from build123d import *

# Parameters (mm, degrees)
SKETCH2_R           = 1.5
SKETCH2_R_2         = 1.6
BOSS_EXTRUDE2_DEPTH = 4.25


with BuildPart() as part:
    # Sketch2 → Boss-Extrude2 (new body)
    with BuildSketch(Plane(origin=(0, 0, 0), x_dir=(1, 0, 0), z_dir=(0, 1, 0))):
        Polygon((184.400116, 296), (225.400116, 255), (241.514718626, 255), (282.514718626, 296), (287.485169777, 296), (291, 292.485169777), (291, 287.514718626), (253, 249.514718626), (253, 226.666961), (291, 188.666961), (291, 181.333039), (253, 143.333039), (253, 120.485281374), (291, 82.485281374), (291, 77.514830223), (287.485169777, 74), (282.514718626, 74), (241.514718626, 115), (225.400116, 115), (184.400116, 74), (175.599884, 74), (134.599884, 115), (113.485281374, 115), (72.485281374, 74), (67.514830223, 74), (64, 77.514830223), (64, 82.485281374), (91, 109.485281374), (91, 123), (81.5, 132.5), (81.5, 163.760895), (64, 181.260895), (64, 188.739105), (81.5, 206.239105), (81.5, 237.5), (91, 247), (91, 260.514718626), (64, 287.514718626), (64, 292.485169777), (67.514830223, 296), (72.485281374, 296), (113.485281374, 255), (134.599884, 255), (175.599884, 296), align=None)
        with Locations(Location((180, 80, 0), (0, 0, 270))):
            Circle(SKETCH2_R, mode=Mode.SUBTRACT)
        with Locations(Location((180, 290, 0), (0, 0, 270))):
            Circle(SKETCH2_R, mode=Mode.SUBTRACT)
        with Locations(Location((285, 80, 0), (0, 0, 270))):
            Circle(SKETCH2_R, mode=Mode.SUBTRACT)
        with Locations(Location((70, 290, 0), (0, 0, 270))):
            Circle(SKETCH2_R, mode=Mode.SUBTRACT)
        with Locations(Location((285, 290, 0), (0, 0, 270))):
            Circle(SKETCH2_R, mode=Mode.SUBTRACT)
        with Locations(Location((70, 185, 0), (0, 0, 270))):
            Circle(SKETCH2_R, mode=Mode.SUBTRACT)
        with Locations(Location((180, 185, 0), (0, 0, 270))):
            Circle(SKETCH2_R, mode=Mode.SUBTRACT)
        with Locations(Location((285, 185, 0), (0, 0, 270))):
            Circle(SKETCH2_R, mode=Mode.SUBTRACT)
        with Locations(Location((256.5, 185, 0), (0, 0, 270))):
            Circle(SKETCH2_R_2, mode=Mode.SUBTRACT)
        with Locations(Location((276.5, 185, 0), (0, 0, 270))):
            Circle(SKETCH2_R_2, mode=Mode.SUBTRACT)
        with Locations(Location((106.5, 220, 0), (0, 0, 270))):
            Circle(SKETCH2_R_2, mode=Mode.SUBTRACT)
        with Locations(Location((106.5, 150, 0), (0, 0, 270))):
            Circle(SKETCH2_R_2, mode=Mode.SUBTRACT)
        with Locations(Location((86.5, 220, 0), (0, 0, 270))):
            Circle(SKETCH2_R_2, mode=Mode.SUBTRACT)
        with Locations(Location((86.5, 150, 0), (0, 0, 270))):
            Circle(SKETCH2_R_2, mode=Mode.SUBTRACT)
        with Locations(Location((70, 80, 0), (0, 0, 270))):
            Circle(SKETCH2_R, mode=Mode.SUBTRACT)
        with Locations(Location((181.5, 165.5, 0), (0, 0, 270))):
            Circle(SKETCH2_R, mode=Mode.SUBTRACT)
        with Locations(Location((181.5, 204.5, 0), (0, 0, 270))):
            Circle(SKETCH2_R, mode=Mode.SUBTRACT)
        Polygon((162, 177.02296782), (141.97703218, 157), (124.999970007, 157), (101.5, 180.5), (101.5, 189.5), (124.999970007, 213), (141.97703218, 213), (162, 192.97703218), align=None, mode=Mode.SUBTRACT)
        Polygon((251.5, 210.014709), (240.98529, 220.529449), (224.014709, 220.529449), (197, 193.51474), (197, 176.48526), (224.014709, 149.470551), (240.98529, 149.470551), (251.5, 159.985291), align=None, mode=Mode.SUBTRACT)
        Polygon((143, 246.415771), (143, 229.566314), (159.566314, 213), (199.51474, 213), (216, 229.48526), (216, 247.429580116), (183.682617, 279.746963116), (176.317383, 279.733154), align=None, mode=Mode.SUBTRACT)
        Polygon((143, 123.584229), (143, 140.433686), (159.566314, 157), (199.51474, 157), (216, 140.51474), (216, 122.570419884), (183.682617, 90.253036884), (176.317383, 90.266846), align=None, mode=Mode.SUBTRACT)
        with BuildLine():
            Line((101.500000013, 226.75), (101.500000013, 213.25))
            Line((101.500000013, 213.25), (102.000000013, 212.75))
            Line((102.000000013, 212.75), (102.100000157, 212.75))
            ThreePointArc((102.100000157, 212.75), (105.1, 209.75), (102.100000157, 206.75))
            Line((102.100000157, 206.75), (90.899999843, 206.75))
            ThreePointArc((90.899999843, 206.75), (87.9, 209.75), (90.899999843, 212.75))
            Line((90.899999843, 212.75), (90.999999987, 212.75))
            Line((90.999999987, 212.75), (91.499999987, 213.25))
            Line((91.499999987, 213.25), (91.499999987, 226.75))
            Line((91.499999987, 226.75), (90.999999987, 227.25))
            Line((90.999999987, 227.25), (90.899999843, 227.25))
            ThreePointArc((90.899999843, 227.25), (87.9, 230.25), (90.899999843, 233.25))
            Line((90.899999843, 233.25), (102.100000157, 233.25))
            ThreePointArc((102.100000157, 233.25), (105.100000157, 230.25), (102.100000157, 227.25))
            Line((102.100000157, 227.25), (102.000000013, 227.25))
            Line((102.000000013, 227.25), (101.500000013, 226.75))
        make_face(mode=Mode.SUBTRACT)
        with BuildLine():
            Line((271.500000013, 191.75), (271.500000013, 178.25))
            Line((271.500000013, 178.25), (272.000000013, 177.75))
            Line((272.000000013, 177.75), (272.100000157, 177.75))
            ThreePointArc((272.100000157, 177.75), (275.100000157, 174.75), (272.100000157, 171.75))
            Line((272.100000157, 171.75), (260.899999843, 171.75))
            ThreePointArc((260.899999843, 171.75), (257.9, 174.75), (260.899999843, 177.75))
            Line((260.899999843, 177.75), (260.999999987, 177.75))
            Line((260.999999987, 177.75), (261.499999987, 178.25))
            Line((261.499999987, 178.25), (261.499999987, 191.75))
            Line((261.499999987, 191.75), (260.999999987, 192.25))
            Line((260.999999987, 192.25), (260.899999843, 192.25))
            ThreePointArc((260.899999843, 192.25), (257.9, 195.25), (260.899999843, 198.25))
            Line((260.899999843, 198.25), (272.100000157, 198.25))
            ThreePointArc((272.100000157, 198.25), (275.100000157, 195.25), (272.100000157, 192.25))
            Line((272.100000157, 192.25), (272.000000013, 192.25))
            Line((272.000000013, 192.25), (271.500000013, 191.75))
        make_face(mode=Mode.SUBTRACT)
        with BuildLine():
            Line((101.500000013, 156.75), (101.500000013, 143.25))
            Line((101.500000013, 143.25), (102.000000013, 142.75))
            Line((102.000000013, 142.75), (102.100000157, 142.75))
            ThreePointArc((102.100000157, 142.75), (105.1, 139.75), (102.100000157, 136.75))
            Line((102.100000157, 136.75), (90.899999843, 136.75))
            ThreePointArc((90.899999843, 136.75), (87.9, 139.75), (90.899999843, 142.75))
            Line((90.899999843, 142.75), (90.999999987, 142.75))
            Line((90.999999987, 142.75), (91.499999987, 143.25))
            Line((91.499999987, 143.25), (91.499999987, 156.75))
            Line((91.499999987, 156.75), (90.999999987, 157.25))
            Line((90.999999987, 157.25), (90.899999843, 157.25))
            ThreePointArc((90.899999843, 157.25), (87.9, 160.25), (90.899999843, 163.25))
            Line((90.899999843, 163.25), (102.100000157, 163.25))
            ThreePointArc((102.100000157, 163.25), (105.100000157, 160.25), (102.100000157, 157.25))
            Line((102.100000157, 157.25), (102.000000013, 157.25))
            Line((102.000000013, 157.25), (101.500000013, 156.75))
        make_face(mode=Mode.SUBTRACT)
    extrude(amount=BOSS_EXTRUDE2_DEPTH)


solid = part.part
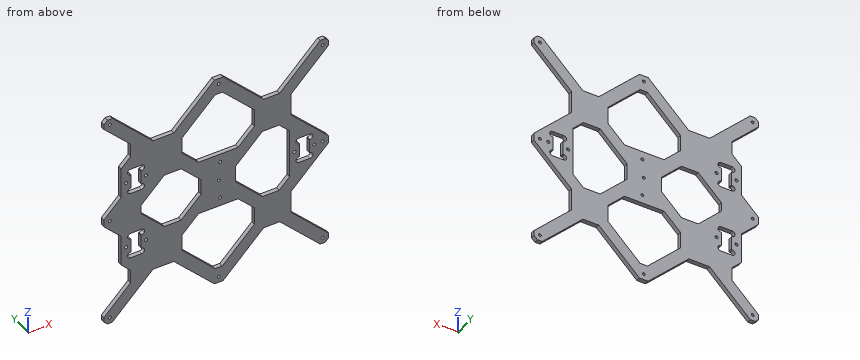
Can you work these out from the model? Positions are in its coordinate system, mm. Round coordinates to 2 decimals unless told otherwise and drop trailing zeros. Loops run counter-clockwise (first coordinate to the right, second up) from the corner with the lowest first, then second, coordinate; pieces in that order, holes last. Notation, with made-up numbers: (4.5, -22.5) - (38.5, -22.5) arc R33 ccw to (38.5, 8.5) - close; hole circle Ø8 at (49, 84.25). An arc over 180 degrees is marked (long way). Use CSV: the item, a comma, the result in double quotes. Start each with the question number.
1) For pin 1 Ø1.3 at (x, y) = (126.5, 1.5) entering from +Z; pin 2 Ø1.5 at (x, y) = (207, 3) entering from +Z; pin 3 Ø1.3 at (y, z) = (2, -147) entering from +X, each with a flat end and sliding along its axis, tell me the tip position at first contact or that it passes through.
2) If we section it at A-A on x = 212: Write out the boundary of the cut face in (y, z), plus the area to 3 significant figures.
3) Please list where these lines run through material, in increasing order: probe 1 along X at (y, z) = (3.35, -236); probe 2 along X at (y, z) = (1.5, -279.5); probe 3 along Z at (x, y) = (281.5, 0.5). Write a range as [from, to].
4) If we section it at C-C on y = 1.9: Count the separate pieces of the cut face and the enclosed holes in it, plus the area to 3 significant figures.
5) If we section it at B-B on z = -103.5: Write out the boundary of the cut face in (x, y), plus the area to 3 significant figures.
Geometry results:
1,pin 1,"stops at z = -115"
1,pin 2,"stops at z = -95.85"
1,pin 3,"stops at x = 257.32"
2,outline,"(0, -268.4) - (4.25, -268.4) - (4.25, -251.43) - (0, -251.43) - close; (0, -225.49) - (4.25, -225.49) - (4.25, -208.51) - (0, -208.51) - close; (0, -161.49) - (4.25, -161.49) - (4.25, -144.51) - (0, -144.51) - close; (0, -118.57) - (4.25, -118.57) - (4.25, -101.6) - (0, -101.6) - close"
2,area,"288 mm2"
3,probe 1,"x = [81.5, 143], [216, 253]"
3,probe 2,"x = [72.01, 88.99], [159.1, 176.08], [183.93, 200.9], [266.01, 282.99]"
3,probe 3,"z = [-294.99, -278.01], [-198.17, -171.83], [-91.99, -75.01]"
4,separate pieces,"1"
4,enclosed holes,"24"
4,area,"19,000 mm2"
5,outline,"(85.01, 0) - (101.99, 0) - (101.99, 4.25) - (85.01, 4.25) - close; (146.1, 0) - (163.08, 0) - (163.08, 4.25) - (146.1, 4.25) - close; (196.93, 0) - (213.9, 0) - (213.9, 4.25) - (196.93, 4.25) - close; (253.01, 0) - (269.99, 0) - (269.99, 4.25) - (253.01, 4.25) - close"
5,area,"289 mm2"
